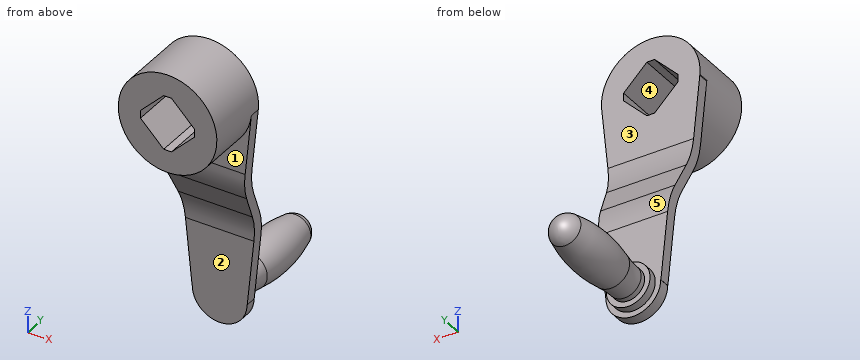
from build123d import *

# Parameters (mm, degrees)
IZIM2_R                     = 45
Y_KSEKLIK_EKSTR_ZYON1_DEPTH = 60
KES_EKSTR_ZYON1_DEPTH       = 61
Y_KSEKLIK_EKSTR_ZYON2_DEPTH = 45
KES_EKSTR_ZYON2_DEPTH       = 61
KES_EKSTR_ZYON4_DEPTH       = 102.850872841
Y_KSEKLIK_EKSTR_ZYON3_DEPTH = 10
IZIM10_R                    = 20
Y_KSEKLIK_EKSTR_ZYON4_DEPTH = 7.5


with BuildPart() as part:
    # Çizim2 → Yükseklik-Ekstrüzyon1 (new body)
    with BuildSketch(Plane(origin=(0, 0, 0), x_dir=(1, 0, 0), z_dir=(0, 1, 0))):
        Circle(IZIM2_R)
    extrude(amount=-Y_KSEKLIK_EKSTR_ZYON1_DEPTH)

    # Çizim5 → Kes-Ekstrüzyon1 (cut, through all)
    with BuildSketch(Plane(origin=(0, 0, 0), x_dir=(1, 0, 0), z_dir=(0, 1, 0))):
        Polygon((-24.748737342, 3.535533906), (-3.535533906, 24.748737342), (3.535533906, 24.748737342), (24.748737342, 3.535533906), (24.748737342, -3.535533906), (3.535533906, -24.748737342), (-3.535533906, -24.748737342), (-24.748737342, -3.535533906), align=None)
    extrude(amount=-KES_EKSTR_ZYON1_DEPTH, mode=Mode.SUBTRACT)

    # Çizim6 → Yükseklik-Ekstrüzyon2 (add, symmetric)
    with BuildSketch(Plane(origin=(0, 0, 0), x_dir=(0, 0, -1), z_dir=(1, 0, 0))):
        with BuildLine():
            Line((60.83592135, 0), (3.535533906, 0))
            Line((3.535533906, 0), (3.535533906, -10))
            Line((3.535533906, -10), (60.83592135, -10))
            ThreePointArc((60.83592135, -10), (74.621096583, -8.394939368), (87.66873708, -3.66563146))
            Line((87.66873708, -3.66563146), (112.33126292, 8.66563146))
            ThreePointArc((112.33126292, 8.66563146), (125.378903417, 13.394939368), (139.16407865, 15))
            Line((139.16407865, 15), (200, 15))
            Line((200, 15), (200, 25))
            Line((200, 25), (139.16407865, 25))
            ThreePointArc((139.16407865, 25), (125.378903417, 23.394939368), (112.33126292, 18.66563146))
            Line((112.33126292, 18.66563146), (87.66873708, 6.33436854))
            ThreePointArc((87.66873708, 6.33436854), (74.621096583, 1.605060632), (60.83592135, 0))
        make_face()
    extrude(amount=Y_KSEKLIK_EKSTR_ZYON2_DEPTH, both=True)

    # Çizim5<2> → Kes-Ekstrüzyon2 (cut, through all)
    with BuildSketch(Plane(origin=(0, 0, 0), x_dir=(1, 0, 0), z_dir=(0, 1, 0))):
        Polygon((-24.748737342, 3.535533906), (-3.535533906, 24.748737342), (3.535533906, 24.748737342), (24.748737342, 3.535533906), (24.748737342, -3.535533906), (3.535533906, -24.748737342), (-3.535533906, -24.748737342), (-24.748737342, -3.535533906), align=None)
    extrude(amount=-KES_EKSTR_ZYON2_DEPTH, mode=Mode.SUBTRACT)

    # Çizim7 → Kes-Ekstrüzyon4 (cut, through all)
    with BuildSketch(Plane(origin=(0, 41.850872841, 0), x_dir=(1, 0, 0), z_dir=(0, 1, 0))):
        with BuildLine():
            ThreePointArc((-45, 0), (-44.94357329, 2.252824878), (-44.77443467, 4.5))
            Line((-44.77443467, 4.5), (-25.125945381, 200))
            Line((-25.125945381, 200), (-45, 200))
            Line((-45, 200), (-45, 0))
        make_face()
        with BuildLine():
            Line((25.125945381, 200), (44.77443467, 4.5))
            ThreePointArc((44.77443467, 4.5), (44.94357329, 2.252824878), (45, 0))
            Line((45, 0), (45, 200))
            Line((45, 200), (25.125945381, 200))
        make_face()
    extrude(amount=-KES_EKSTR_ZYON4_DEPTH, mode=Mode.SUBTRACT)

    # Çizim9 → Yükseklik-Ekstrüzyon3 (add)
    with BuildSketch(Plane(origin=(0, 25, 0), x_dir=(1, 0, 0), z_dir=(0, 1, 0))):
        with BuildLine():
            Line((-25, 200), (25, 200))
            ThreePointArc((25, 200), (0, 225), (-25, 200))
        make_face()
    extrude(amount=-Y_KSEKLIK_EKSTR_ZYON3_DEPTH)

    # Çizim10 → Yükseklik-Ekstrüzyon4 (add)
    with BuildSketch(Plane(origin=(0, 25, 0), x_dir=(1, 0, 0), z_dir=(0, 1, 0))):
        with Locations((0, 200)):
            Circle(IZIM10_R)
    extrude(amount=Y_KSEKLIK_EKSTR_ZYON4_DEPTH)

    # Çizim12 → Döndür5 (revolve)
    with BuildSketch(Plane(origin=(0, 0, 0), x_dir=(0, 0, -1), z_dir=(1, 0, 0))):
        with BuildLine():
            ThreePointArc((214.501915582, 123.333333333), (209.151502609, 131.384864324), (200, 134.5))
            Line((200, 134.5), (200, 119.5))
            Line((200, 119.5), (200, 32.5))
            Line((200, 32.5), (215, 32.5))
            Line((215, 32.5), (215, 37.5))
            ThreePointArc((215, 37.5), (215.45962104, 47.262068061), (216.83441772, 56.937767437))
            ThreePointArc((216.83441772, 56.937767437), (219.390284523, 90.266309839), (214.501915582, 123.333333333))
        make_face()
    revolve(axis=Axis((0, 25, -200), (0, 1, 0)))


solid = part.part
The listing builds one solid part. Answer for the finished solid, in the listing's coordinates (mm). Face numbers are marked on the shaded views. A direction names the side the tool comes from. Round coordinates to 2 decimals unless told otherwise and drop trailing zeros. Write each loop counter-clockwise with the first axis right and the second up, starting at its lowest first coordinate (ties: lowest second). Pieces come first, ordered by that corner, then holes. Notation, with made-up numbers: (59.25, -35.75) - (104.25, -35.75) arc R15 ccw to (104.25, -24.75) - close; hole circle Ø11 at (73.5, 59.25). An arc over 180 degrees is marked (long way). Use a Markdown table: item, result. Add a question column.
1. A tool of negligible diameter and unlimited length cuts with its end or side. For the marked faces 1, 2 and 3, from which of +Z, -Z, +X, -X, +Y, -Y can it reach the whole face along a straight path? Write none if from no direction.
2. The part is cut by section B-B (y = -47). Write down the section's boundary in (x, z).
3. Flat-ended cylindrical pins translate along their axes: P1, Ø1.5, axis at y = 103.5, z = -196.5, coming from the -X side; P2, Ø2, axis at x = -1.5, y = -39, coming from the +Z side; P3, Ø18.5, axis at x = 1.5, z = -179, coming from the +Y side. Find the tip coordinate at first contact, or state that the pin passes through.
4. The part is cut by section A-A (z = 0). Write down the section's boundary in (x, y).
5. The part is cut by section D-D (z = -117). Write down the section's boundary in (x, y), and give its area (3 significant figures).
6. For a pull along X with two mould halves and no side action, classify the marked faces 4 and 5 as +X half, -X half, draft (parallel to the pull), parting line (faces both ways), or undercut.
7. Consider line 1 (Y direction, x = -29, z = -145); line 2 (Z direction, x = 5, y = -52); line 3 (Z direction, x = -20.5, y = -5.5). Determine where each line is inside the solid, lowest interval first.
8. The part is cut by section C-C (z = -40.5). Write down the section's boundary in (x, y), and give its area (3 significant figures).
Reported:
| question | item | result |
|---|---|---|
| 1 | face 1 | -Z, -Y |
| 1 | face 2 | -Z, +X, -X, -Y |
| 1 | face 3 | +Z, +X, -X, +Y |
| 2 | outline | circle Ø90 at (0, 0); hole (-24.75, -3.54) - (-3.54, -24.75) - (3.54, -24.75) - (24.75, -3.54) - (24.75, 3.54) - (3.54, 24.75) - (-3.54, 24.75) - (-24.75, 3.54) - close |
| 3 | P1 | x = -18.16 |
| 3 | P2 | z = 45 |
| 3 | P3 | y = 128.76 |
| 4 | outline | (-45, -60) - (-24.75, -60) - (-24.75, 0) - (-45, 0) - close; (24.75, -60) - (45, -60) - (45, 0) - (24.75, 0) - close |
| 5 | outline | (-33.47, 10.76) - (33.47, 10.76) - (33.47, 20.76) - (-33.47, 20.76) - close |
| 5 | area | 669 mm^2 |
| 6 | face 4 | undercut |
| 6 | face 5 | draft |
| 7 | line 1 | 15 to 25 |
| 7 | line 2 | -44.72 to -23.28, 23.28 to 44.72 |
| 7 | line 3 | -83.63 to -7.78, 7.78 to 40.06 |
| 8 | outline | (-41.16, -10) - (-19.62, -10) - (-19.62, -60) - (19.62, -60) - (19.62, -10) - (41.16, -10) - (41.16, 0) - (-41.16, 0) - close |
| 8 | area | 2,780 mm^2 |
